Read the model definition and answer for the solid it produces. Units are mm, in the model's axes. A direction names the side the tool comes from. Give positions to 0.01 mm unless a question says otherwise; leave off trailing zeros. Loops run counter-clockwise (first coordinate to the right, second up) from the corner with the lowest first, then second, coordinate; pieces in that order, holes last. Notation, with made-up numbers: (20.5, 73.25) -> (75.5, 73.25) arc R14 ccw to (75.5, 100.25) -> close; hole circle Ø2 at (40.25, -35). An arc over 180 degrees is marked (long way). Return JSON: item names as keys, results as strings. Group by question number.
from build123d import *

# Parameters (mm, degrees)
SKETCH_1_W          = 125.74675372
SKETCH_1_H          = 106.976622422
EXTRUDE_3_DEPTH     = 30
SKETCH_3_W          = 40.480715441
SKETCH_3_H          = 75.445810288
CUT_EXTRUDE_2_DEPTH = 20
SKETCH_6_W          = 4.561176424
SKETCH_6_H          = 3.413136976
SKETCH_6_W_2        = 27.210286446
SKETCH_6_H_2        = 12.79926366
SKETCH_6_W_3        = 17.507485433
SKETCH_6_H_3        = 32.993657433
CUT_EXTRUDE_6_DEPTH = 20
CUT_EXTRUDE_7_DEPTH = 10
SKETCH_8_W          = 43.362055896
SKETCH_8_H          = 5.90330429
EXTRUDE_4_DEPTH     = 30
SKETCH_9_W          = 43.362055896
SKETCH_9_H          = 30
SKETCH_9_R          = 13.106917469
EXTRUDE_5_DEPTH     = 50


with BuildPart() as part:
    # 草图1 → 凸台-拉伸3 (new body)
    with BuildSketch(Plane.XY):
        Rectangle(SKETCH_1_W, SKETCH_1_H)
    extrude(amount=EXTRUDE_3_DEPTH)

    # 草图3 → 切除-拉伸2 (cut)
    with BuildSketch(Plane.XY):
        with Locations((-0.814646552, -3.347576181)):
            Rectangle(SKETCH_3_W, SKETCH_3_H)
    extrude(amount=CUT_EXTRUDE_2_DEPTH, mode=Mode.SUBTRACT)

    # 草图6 → 切除-拉伸6 (cut)
    with BuildSketch(Plane.XY):
        with Locations((60.592788648, 44.118378059)):
            Rectangle(SKETCH_6_W, SKETCH_6_H)
        with Locations((44.707057213, 43.502117216)):
            Rectangle(SKETCH_6_W_2, SKETCH_6_H_2)
        with Locations((-48.375754904, 33.501377131)):
            Rectangle(SKETCH_6_W_3, SKETCH_6_H_3)
    extrude(amount=CUT_EXTRUDE_6_DEPTH, mode=Mode.SUBTRACT)

    # 草图7 → 切除-拉伸7 (cut)
    with BuildSketch(Plane.XY):
        with BuildLine():
            Line((31.10191399, 49.901749046), (19.425711168, 49.901749046))
            Line((19.425711168, 49.901749046), (18.685275266, 49.901749046))
            ThreePointArc((18.685275266, 49.901749046), (17.978168485, 49.608855827), (17.685275266, 48.901749046))
            Line((17.685275266, 48.901749046), (17.685275266, 34.375328963))
            Line((17.685275266, 34.375328963), (19.425711168, 34.375328963))
            Line((19.425711168, 34.375328963), (19.425711168, 46.90603785))
            ThreePointArc((19.425711168, 46.90603785), (19.718604387, 47.613144632), (20.425711168, 47.90603785))
            Line((20.425711168, 47.90603785), (31.10191399, 47.90603785))
            Line((31.10191399, 47.90603785), (31.10191399, 49.901749046))
        make_face()
        with BuildLine():
            Line((-39.622012187, 17.004548414), (-40.809816648, 17.004548414))
            Line((-40.809816648, 17.004548414), (-40.809816648, 6.183104922))
            Line((-40.809816648, 6.183104922), (-40.809816648, 5.834646341))
            ThreePointArc((-40.809816648, 5.834646341), (-40.516923429, 5.12753956), (-39.809816648, 4.834646341))
            Line((-39.809816648, 4.834646341), (-21.055004273, 4.834646341))
            Line((-21.055004273, 4.834646341), (-21.055004273, 6.183104922))
            Line((-21.055004273, 6.183104922), (-38.622012187, 6.183104922))
            ThreePointArc((-38.622012187, 6.183104922), (-39.329118968, 6.475998141), (-39.622012187, 7.183104922))
            Line((-39.622012187, 7.183104922), (-39.622012187, 17.004548414))
        make_face()
    extrude(amount=CUT_EXTRUDE_7_DEPTH, mode=Mode.SUBTRACT)

    # 草图8 → 凸台-拉伸4 (add)
    with BuildSketch(Plane.XY):
        with Locations((84.554404808, -50.536659066)):
            Rectangle(SKETCH_8_W, SKETCH_8_H)
    extrude(amount=EXTRUDE_4_DEPTH)

    # 草图9 → 凸台-拉伸5 (add)
    with BuildSketch(Plane(origin=(0, 0, 0), x_dir=(1, 0, 0), z_dir=(0, 1, 0))):
        with Locations((84.554404808, -15)):
            Rectangle(SKETCH_9_W, SKETCH_9_H)
        with Locations(Location((84.554404808, -15, 0), (0, 0, 270))):
            Circle(SKETCH_9_R, mode=Mode.SUBTRACT)
    extrude(amount=-EXTRUDE_5_DEPTH)


solid = part.part
1. Section B-B on x = -2.5 is taken. Determine the outline of the cut face in (y, z), then the cut area to 3 significant figures.
2. Section A-A on z = 15 is taken. Determine the outline of the cut face in (x, y) (1 decimal), then the cut area to 3 significant figures.
3. Straight lines are drawn through the part: line 1 (X direction, y = 49.5, z = 17.75); line 2 (X direction, y = 20, z = 15) (1 decimal); line 3 (X direction, y = 10, z = 19.25) (3 decimals). For each, find the intervals that lie inside material, in ascending order. Write a range as from..to.
4. Section C-C on y = 2.5 is taken. Determine the outline of the cut face in (x, z) (3 decimals).
5. Section D-D on z = 25.75 is taken. Determine the outline of the cut face in (x, y) (3 decimals).
6. Determine the mould class of faces 4 (the flat face through (17.685, 42, 5)), 5 (the flat face through (20, -11, 0)) for opening direction X: pulls with the +X half, pulls with the -X half, needs draft (parallel to the pull), parting line crosses it, or undercut.
7. Which of the six approach directions +Z, -Z, +X, -X, +Y, -Y give full straight-line access (tool end or side, diameter ignored) to faces 1 (the flat face through (20, 1, 30)), 2 (the flat face through (84, 0, 1)), 3 (the flat face through (43, 49.902, 10))?
8. Flat-ended cylindrical pins translate along their axes: pin 1 Ø6.5 at (x, y) = (27, 44) entering from -Z; pin 2 Ø15 at (y, z) = (24, 11) entering from +X; pin 3 Ø5.5 at (x, y) = (-48.5, 25.5) entering from -Z. Find the tip coordinate at first contact, or state that the pin passes through.
Completed:
{
 "1": {"outline": "(-53.49, 0) -> (-41.07, 0) -> (-41.07, 20) -> (34.38, 20) -> (34.38, 0) -> (53.49, 0) -> (53.49, 30) -> (-53.49, 30) -> close", "area": "1,700 mm²"},
 "2": {"outline": "(-62.9, -53.5) -> (106.2, -53.5) -> (106.2, 0) -> (97.7, 0) -> (97.7, -47.6) -> (71.4, -47.6) -> (71.4, 0) -> (62.9, 0) -> (62.9, 42.4) -> (58.3, 42.4) -> (58.3, 37.1) -> (31.1, 37.1) -> (31.1, 49.9) -> (58.3, 49.9) -> (58.3, 45.8) -> (62.9, 45.8) -> (62.9, 53.5) -> (-62.9, 53.5) -> close; hole (-57.1, 17) -> (-39.6, 17) -> (-39.6, 50) -> (-57.1, 50) -> close; hole (-21.1, -41.1) -> (19.4, -41.1) -> (19.4, 34.4) -> (-21.1, 34.4) -> close", "area": "10,500 mm²"},
 "3": {"line 1": "x = -62.87..-57.13, -39.62..31.1, 58.31..62.87", "line 2": "x = -62.9..-57.1, -39.6..-21.1, 19.4..62.9", "line 3": "x = -62.873..-21.055, 19.426..62.873"},
 "4": {"outline": "(-62.873, 0) -> (-21.055, 0) -> (-21.055, 20) -> (19.426, 20) -> (19.426, 0) -> (62.873, 0) -> (62.873, 30) -> (-62.873, 30) -> close"},
 "5": {"outline": "(-62.873, -53.488) -> (106.235, -53.488) -> (106.235, 0) -> (92.053, 0) -> (92.053, -47.585) -> (77.056, -47.585) -> (77.056, 0) -> (62.873, 0) -> (62.873, 53.488) -> (-62.873, 53.488) -> close"},
 "6": {"face 4": "undercut", "face 5": "needs draft"},
 "7": {"face 1": "+Z, +X, -X, +Y, -Y", "face 2": "+Z, -Z, +X, +Y", "face 3": "-Z"},
 "8": {"pin 1": "stops at z = 0", "pin 2": "stops at x = 62.87", "pin 3": "stops at z = 20"}
}
